Geometry: final body of the model. Coordinates: model frame, mm. A direction names the side the tool comes from. Round coordinates to 2 decimals unless told otherwise and drop trailing zeros. Write each loop counter-clockwise with the first axis right and the second up, starting at its lowest first coordinate (ties: lowest second). Pieces come first, ordered by that corner, then holes. Notation, with made-up numbers: M -39,86 L -15,86 A14 cw -15,105 Z; hole C 64,88 d4. An arc over 180 degrees is marked long. Put each result on its own line as item: value. Start each with the question number.
```python
from build123d import *

# Parameters (mm, degrees)
F0_W     = 304.8
F0_H     = 203.2
F1_DEPTH = 177.8
F2_T     = -10.16
F3_T     = -0.254


with BuildPart() as f1:
    # F0 (on Top) → F1 (new body)
    with BuildSketch(Plane.XY):
        with Locations((-48.5099423885, -25.4367205143)):
            Rectangle(F0_W, F0_H)
    extrude(amount=F1_DEPTH)

    # F2
    f2_openings = [f1.faces().sort_by_distance(p)[0] for p in [
        (-48.509942, -25.436721, 0),
    ]]
    offset(amount=F2_T, openings=f2_openings)

    # F3
    f3_openings = [f1.faces().sort_by_distance(p)[0] for p in [
        (103.890058, -25.436721, 88.9),
    ]]
    offset(amount=F3_T, openings=f3_openings, kind=Kind.INTERSECTION)


solid = f1.part
```
1) Section B-B, the plane x = 18. Output: boundary loops of the cut face in (y, z).
2) Ray query, probe 1 along X at (y, z) = (-100, 95.5); probe 2 along Y at (x, z) = (-140, 19); probe 3 along Z at (x, y) = (-179.5, -94). Return the intervals inside material, ascending.
3) Draft query along Z for faces 1 (the face through (-51, 76.163, 88)), 2 (the face through (-200.656, -27, 88)), 3 (the face through (-51, -24, 167.64)). Return one class per face: +Z half, -Z half, draft (parallel to the pull), parting line (faces both ways), or undercut.
4) Access query for faces 4 (the face through (-191.004, -27, 83)), 5 (the face through (-51, -116.877, 83)), 6 (the face through (-51, -127.037, 88)), 7 (the face through (-51, -24, 177.546)). Directions: +Z, -Z, +X, -X, +Y, -Y. A direction counts if a zero-diameter tool reaches every point of the face in a straight line with its end or side. Return the directions, or none.
5) Section A-A, the plane z = 103.5. Output: boundary loops of the cut face in (x, y), and give its area (3 significant figures).
6) Section C-C, the plane y = 26. Output: boundary loops of the cut face in (x, z), and give its area (3 significant figures).
7) First-contact query: pin 1 (5 mm diameter, centred on x = 66.5, y = -54, fed in from -Z); pin 2 (8 mm diameter, centred on y = 22.5, z = 68, fed in from +X). Flat tips, straight axial feed; report the tip coordinate or a pass-through.
Solved:
1. outline: M -127.04,0 L -116.88,0 L -116.88,167.64 L 66,167.64 L 66,0 L 76.16,0 L 76.16,177.8 L -127.04,177.8 Z; hole M -126.78,0.25 L -117.13,0.25 L -117.13,167.89 L 66.26,167.89 L 66.26,0.25 L 75.91,0.25 L 75.91,177.55 L -126.78,177.55 Z
2. probe 1: x = -200.91 to -200.66, -191 to -190.75, 93.73 to 93.98
2. probe 2: y = -127.04 to -126.78, -117.13 to -116.88, 66 to 66.26, 75.91 to 76.16
2. probe 3: z = 167.64 to 167.89, 177.55 to 177.8
3. face 1: draft
3. face 2: undercut
3. face 3: -Z half
4. face 4: none
4. face 5: -Z
4. face 6: +Z, -Z, +X, -X, -Y
4. face 7: +X
5. outline: M -200.91,-127.04 L 103.89,-127.04 L 103.89,-126.78 L -200.66,-126.78 L -200.66,75.91 L 103.89,75.91 L 103.89,76.16 L -200.91,76.16 Z; M -191,-117.13 L 93.98,-117.13 L 93.98,66.26 L -191,66.26 Z; hole M -190.75,-116.88 L 93.73,-116.88 L 93.73,66 L -190.75,66 Z
5. area: 444 mm2
6. outline: M -200.91,0 L -190.75,0 L -190.75,167.64 L 93.73,167.64 L 93.73,0 L 103.89,0 L 103.89,0.25 L 93.98,0.25 L 93.98,167.89 L -191,167.89 L -191,0.25 L -200.66,0.25 L -200.66,177.55 L 103.89,177.55 L 103.89,177.8 L -200.91,177.8 Z
6. area: 285 mm2
7. pin 1: stops at z = 167.64
7. pin 2: stops at x = 93.98
